Source: three-view drawing plus pictorial views. Frame: mm from the lowest corner of the part. Give positions to 0.01 mm unless a question says otherwise; leave off trailing zeros. Order: outer loops, then holes, each group sorted by start corner. A loop starts at its lowest first (then second) coordinate and runs counter-clockwise, first axis right, second up. Notation, with made-up numbers: (-13, -13) - (13, -13) arc R23 ccw to (13, 23) - close; hole circle Ø7 at (3.25, 30). An arc over 180 degrees is marked (long way). Use one line per item in the form item = value.
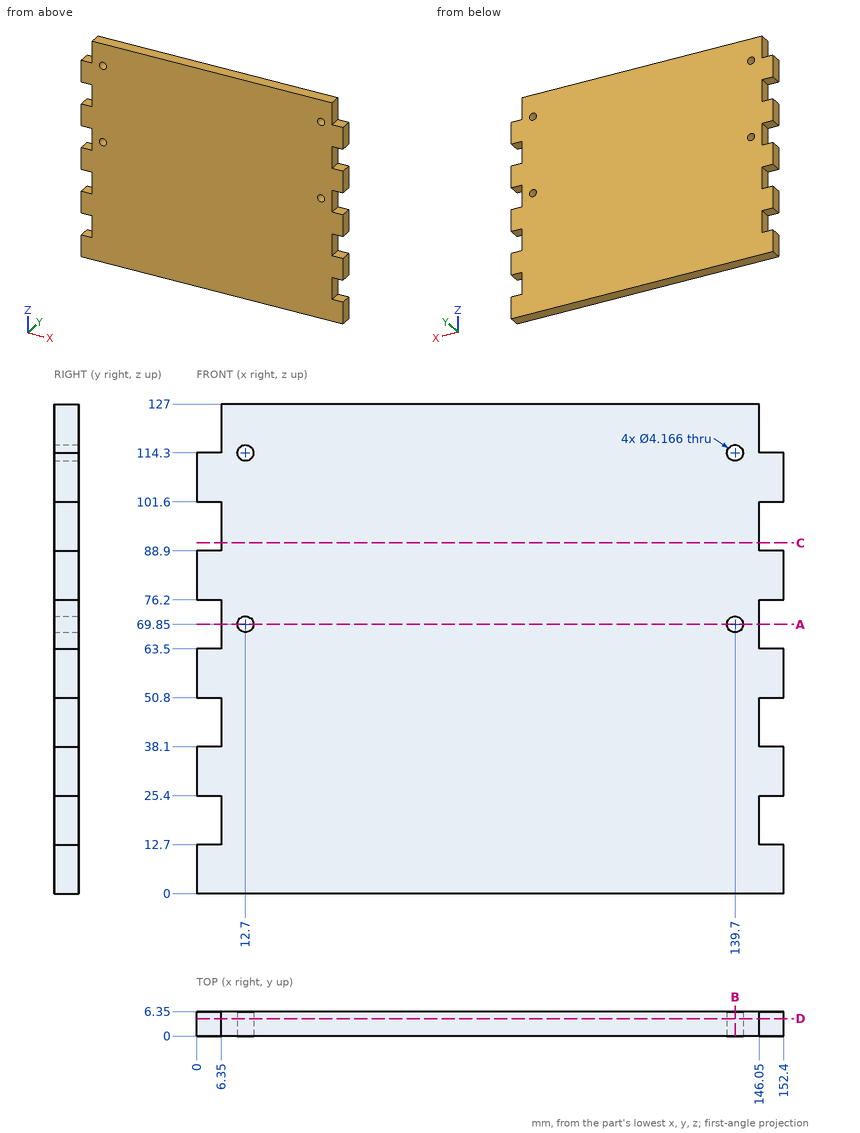
(1) Cut plane B-B on x = 139.7. Output: boundary loops of the cut face in (y, z).
Computed values:
outline = (0, 0) - (6.35, 0) - (6.35, 67.77) - (0, 67.77) - close; (0, 71.93) - (6.35, 71.93) - (6.35, 112.22) - (0, 112.22) - close; (0, 116.38) - (6.35, 116.38) - (6.35, 127) - (0, 127) - close
(2) Cut plane D-D on y = 4.5. Give the number of separate pieces and of enclosed holes in the cut face, plus the area to 3 significant figures.
Computed values:
separate_pieces = 1
enclosed_holes = 4
area = 18,500 mm²
(3) Ray query, line 1 along X through (y, z) = (1.5, 69.85); line 2 along X through (y, z) = (4.5, 38.5). Return the intervals inside material, ascending.
Computed values:
line_1 = 6.35 to 10.62, 14.78 to 137.62, 141.78 to 146.05
line_2 = 6.35 to 146.05
(4) Cut plane A-A on z = 69.85. Output: boundary loops of the cut face in (x, y), plus the area to 3 significant figures.
Computed values:
outline = (6.35, 0) - (10.62, 0) - (10.62, 6.35) - (6.35, 6.35) - close; (14.78, 0) - (137.62, 0) - (137.62, 6.35) - (14.78, 6.35) - close; (141.78, 0) - (146.05, 0) - (146.05, 6.35) - (141.78, 6.35) - close
area = 834 mm²
(5) Contact query for flat-ended pins moving along their axis: pin 1 Ø1.9 at (y, z) = (2.5, 44) entering from +X; pin 2 Ø3.5 at (x, z) = (12.7, 69.85) entering from +Y; pin 3 Ø1.9 at (x, y) = (148.5, 2.5) entering from +Z. Output: stop coordinate, or through.
Computed values:
pin_1 = 146.05
pin_2 = through
pin_3 = 114.3
(6) Cut plane C-C on z = 91. Output: boundary loops of the cut face in (x, y).
Computed values:
outline = (6.35, 0) - (146.05, 0) - (146.05, 6.35) - (6.35, 6.35) - close
